Geometry check sheet. Reference: drawing and pictorial views, mm from the part's lowest x, y, z. Coordinates: 2 decimals unless noted, no trailing zeros. Write each loop counter-clockwise with the first axis right and the second up, starting at its lowest first coordinate (ties: lowest second). Pieces come first, ordered by that corner, then holes. Notation, with made-up numbers: M 70,55 L 85,55 A22 cw 85,67 Z; hole C 40,1.5 d11. An arc over 180 degrees is marked long. One line per item, written item: value.
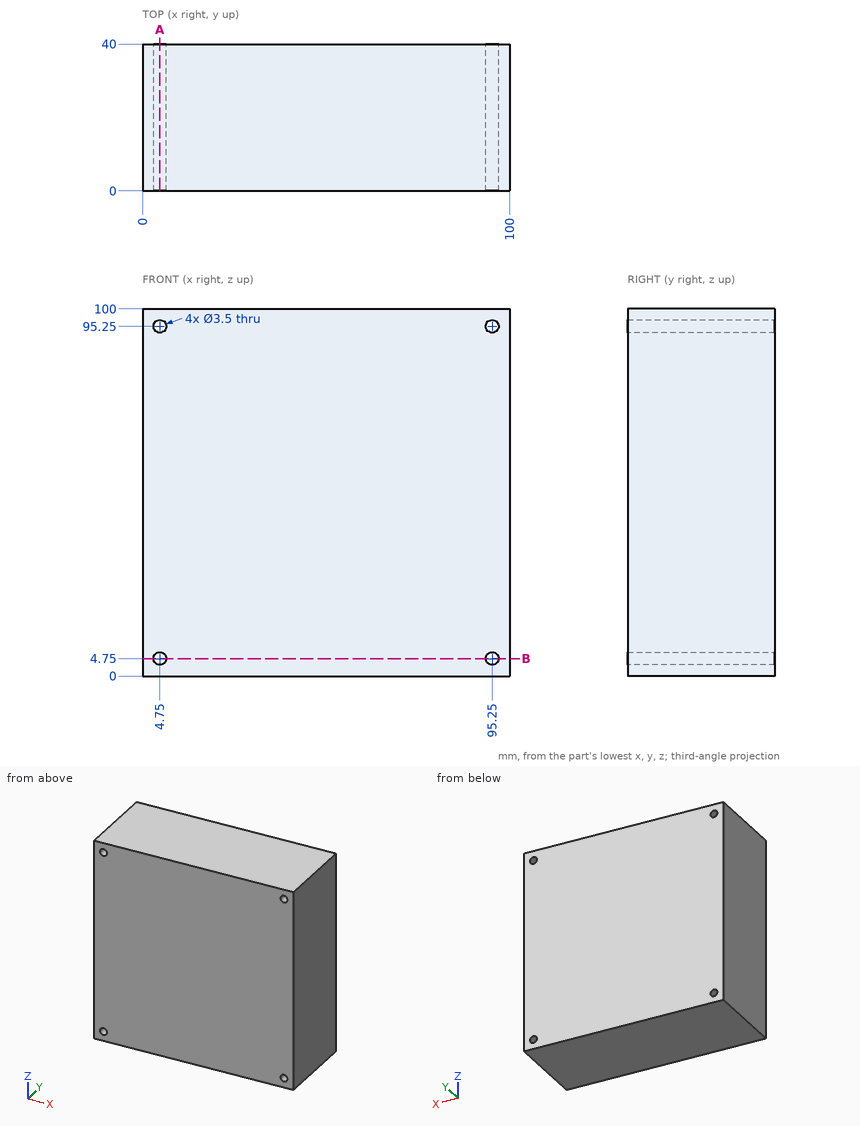
Item 1: Cross-section at A-A, the plane x = 4.75. Enter the section's corners in (y, z), and give its area (3 significant figures).
The answers:
outline: M 0,0 L 40,0 L 40,3 L 0,3 Z; M 0,6.5 L 40,6.5 L 40,93.5 L 0,93.5 Z; M 0,97 L 40,97 L 40,100 L 0,100 Z
area: 3,720 mm²
Item 2: Scan lines: line 1 (Z direction, x = 95.25, y = 19.5); line 2 (X direction, y = 13, z = 4). Record each from-to range of solid material in increasing order.
The answers:
line 1: z = 0 to 3, 6.5 to 93.5, 97 to 100
line 2: x = 0 to 3.17, 6.33 to 93.67, 96.83 to 100
Item 3: Go/stop test with a flat-tipped pin: P1, Ø4, axis at x = 95.25, z = 4.75, coming from the -Y side. Record where the tip stops, or that it passes through.
The answers:
P1: stops at y = 0
Item 4: Cross-section at B-B, the plane z = 4.75. Enter the section's corners in (x, y).
The answers:
outline: M 0,0 L 3,0 L 3,40 L 0,40 Z; M 6.5,0 L 93.5,0 L 93.5,40 L 6.5,40 Z; M 97,0 L 100,0 L 100,40 L 97,40 Z
